from build123d import *

# Parameters (mm, degrees)
BOSS_EXTRUDE1_DEPTH        = 3.175
F_1_0_228_DIAMETER_HOLE2_D = 5.7912
FILLET2_R                  = 2.54
CUT_EXTRUDE3_OUTLINE_R     = 2.8956
CUT_EXTRUDE3_OUTLINE_R_2   = 19.05
CUT_EXTRUDE3_DEPTH         = 3.175


# Read off the part's stored shape, not the designer's step: Cut-Extrude3
with BuildPart() as part:
    # Sketch1 → Boss-Extrude1 (new body)
    with BuildSketch(Plane(origin=(0, 0, 0), x_dir=(1, 0, 0), z_dir=(0, 1, 0))):
        with BuildLine():
            Line((337.058, 219.456), (337.058, 273.558))
            Line((337.058, 273.558), (-337.058, 273.558))
            Line((-337.058, 273.558), (-337.058, -273.558))
            Line((-337.058, -273.558), (337.058, -273.558))
            Line((337.058, -273.558), (337.058, -218.948))
            ThreePointArc((337.058, -218.948), (327.406, -209.296), (337.058, -199.644))
            Line((337.058, -199.644), (337.058, -9.398))
            ThreePointArc((337.058, -9.398), (346.71, 0.254), (337.058, 9.906))
            Line((337.058, 9.906), (337.058, 200.152))
            ThreePointArc((337.058, 200.152), (327.406, 209.804), (337.058, 219.456))
        make_face()
    extrude(amount=BOSS_EXTRUDE1_DEPTH)

    # #1 (0.228) Diameter Hole2 (through all)
    with Locations(Plane(origin=(0, 3.175, 0), x_dir=(1, 0, 0), z_dir=(0, 1, 0))):
        with Locations((337.058, 0.254)):
            Hole(F_1_0_228_DIAMETER_HOLE2_D / 2)

    # Fillet2
    fillet2_edges = [part.edges().sort_by_distance(p)[0] for p in [
        (337.058, 1.5875, -273.558),
        (337.058, 1.5875, -219.456),
        (337.058, 1.5875, -200.152),
        (337.058, 1.5875, -9.906),
        (337.058, 1.5875, 9.398),
        (337.058, 1.5875, 199.644),
        (337.058, 1.5875, 218.948),
        (337.058, 1.5875, 273.558),
        (-337.058, 1.5875, 273.558),
        (-337.058, 1.5875, -273.558),
    ]]
    fillet(fillet2_edges, radius=FILLET2_R)

    # Cut-Extrude3 outline → Cut-Extrude3 (cut)
    with BuildSketch(Plane(origin=(0, 0, 0), x_dir=(1, 0, 0), z_dir=(0, 1, 0))):
        with Locations((284.226, -263.398)):
            Circle(CUT_EXTRUDE3_OUTLINE_R)
        with Locations((4.826, -263.398)):
            Circle(CUT_EXTRUDE3_OUTLINE_R)
        with Locations((-274.574, -263.398)):
            Circle(CUT_EXTRUDE3_OUTLINE_R)
        with Locations((-327.406, -209.296)):
            Circle(CUT_EXTRUDE3_OUTLINE_R)
        with Locations((-327.406, 0.254)):
            Circle(CUT_EXTRUDE3_OUTLINE_R)
        with Locations((-327.406, 209.804)):
            Circle(CUT_EXTRUDE3_OUTLINE_R)
        with Locations((-274.574, 263.906)):
            Circle(CUT_EXTRUDE3_OUTLINE_R)
        with Locations((4.826, 263.906)):
            Circle(CUT_EXTRUDE3_OUTLINE_R)
        with Locations((284.226, 263.906)):
            Circle(CUT_EXTRUDE3_OUTLINE_R)
        with Locations((-260.858, -197.358)):
            Circle(CUT_EXTRUDE3_OUTLINE_R_2)
    extrude(amount=CUT_EXTRUDE3_DEPTH, mode=Mode.SUBTRACT)


solid = part.part
Work out the finished part from the listing and answer in its coordinate system (mm). Coordinates: 2 decimals unless noted, no trailing zeros.
1. The part is cut by section A-A, the plane y = 2. State how many separate pieces and enclosed holes the cut face has, and give its area (3 significant figures).
Results list:
separate pieces: 1
enclosed holes: 11
area: 367,000 mm2
2. A flat-ended cylindrical pin translates along its axis: pin 1 (1.6 mm diameter, centred on y = 1.5, z = 236.5, fed in from +X). Find the tip coordinate at first contact, or state that the pin passes through.
Results list:
pin 1: stops at x = 337.06
3. For a pull along Z with two mould halves and no side action, classify faces 1 (the cylindrical face through (-243.26, 1.57, 204.65)), 2 (the flat face through (0, 3.175, -4)) as +Z half, -Z half, draft (parallel to the pull), parting line (faces both ways), or undercut.
Results list:
face 1: undercut
face 2: draft
4. Consider line 1 along Z through (x, y) = (-259, 1.7); line 2 along X through (y, z) = (0.25, -42.5); line 3 along X through (y, z) = (1.05, -7). Determine where each line is inside the solid, lowest interval first.
Results list:
line 1: z = -273.56 to 178.4, 216.32 to 273.56
line 2: x = -337.06 to 337.06
line 3: x = -337.06 to 343.96
